```python
from build123d import *

# Parameters (mm, degrees)
SZKIC1_W                     = 100
SZKIC1_H                     = 100
DODANIE_WYCI_GNI_CIE1_DEPTH  = 40
SZKIC3_R                     = 22.5
WYTNIJ_WYCI_GNI_CIE1_DEPTH   = 41
SZKIC4_W                     = 100
SZKIC4_H                     = 10
DODANIE_WYCI_GNI_CIE2_DEPTH  = 30
DODANIE_WYCI_GNI_CIE3_DEPTH  = 10
DODANIE_WYCI_GNI_CIE4_DEPTH  = 10
DODANIE_WYCI_GNI_CIE5_DEPTH  = 10
SZKIC11_W                    = 15
SZKIC11_H                    = 50
DODANIE_WYCI_GNI_CIE6_DEPTH  = 70
SZKIC12_R                    = 15
DODANIE_WYCI_GNI_CIE7_DEPTH  = 125
SZKIC13_R                    = 15
DODANIE_WYCI_GNI_CIE8_DEPTH  = 30
DODANIE_WYCI_GNI_CIE9_DEPTH  = 10
ZAOKR_GLENIE1_R              = 20
SZKIC15_W                    = 50
SZKIC15_H                    = 185
DODANIE_WYCI_GNI_CIE10_DEPTH = 10
DODANIE_WYCI_GNI_CIE11_REACH = 52
SZKIC17_W                    = 50
SZKIC17_H                    = 30
SZKIC18_W                    = 100
SZKIC18_H                    = 100
DODANIE_WYCI_GNI_CIE12_DEPTH = 10
DODANIE_WYCI_GNI_CIE13_DEPTH = 10
WYTNIJ_WYCI_GNI_CIE2_REACH   = 202
SZKIC20_R                    = 5
SZKIC21_W                    = 10
SZKIC21_H                    = 25
DODANIE_WYCI_GNI_CIE14_DEPTH = 25
ZAOKR_GLENIE2_R              = 10
WYTNIJ_WYCI_GNI_CIE3_REACH   = 32
SZKIC22_R                    = 5


with BuildPart() as part:
    # Szkic1 → Dodanie-wyciągnięcie1 (new body)
    with BuildSketch(Plane.XY):
        Rectangle(SZKIC1_W, SZKIC1_H)
    extrude(amount=DODANIE_WYCI_GNI_CIE1_DEPTH)

    # Szkic3 → Wytnij-wyciągnięcie1 (cut, through all)
    with BuildSketch(Plane.XY.offset(40)):
        Circle(SZKIC3_R)
    extrude(amount=-WYTNIJ_WYCI_GNI_CIE1_DEPTH, mode=Mode.SUBTRACT)

    # Szkic4 → Dodanie-wyciągnięcie2 (add)
    with BuildSketch(Plane(origin=(0, 0, 0), x_dir=(-1, 0, 0), z_dir=(0, 0, -1))):
        with Locations((0, -45)):
            Rectangle(SZKIC4_W, SZKIC4_H)
    extrude(amount=DODANIE_WYCI_GNI_CIE2_DEPTH)

    # Szkic5 → Dodanie-wyciągnięcie3 (add)
    with BuildSketch(Plane.ZY.offset(50)):
        Polygon((-30, -40), (-250, 50), (0, 50), (0, -40), align=None)
    extrude(amount=-DODANIE_WYCI_GNI_CIE3_DEPTH)

    # Szkic6 → Dodanie-wyciągnięcie4 (add)
    with BuildSketch(Plane(origin=(50, 0, 0), x_dir=(0, 0, -1), z_dir=(1, 0, 0))):
        Polygon((30, -40), (250, 50), (0, 50), (0, -40), align=None)
    extrude(amount=-DODANIE_WYCI_GNI_CIE4_DEPTH)

    # Szkic7 → Dodanie-wyciągnięcie5 (add)
    with BuildSketch(Plane(origin=(0, 50, 0), x_dir=(1, 0, 0), z_dir=(0, 1, 0))):
        Polygon((40, 250), (-40, 250), (-40, 30), (-40, 0), (40, 0), align=None)
    extrude(amount=-DODANIE_WYCI_GNI_CIE5_DEPTH)

    # Szkic10 → Obrót1 (revolve)
    with BuildSketch(Plane(origin=(0, 0, -200), x_dir=(-1, 0, 0), z_dir=(0, 0, -1))):
        Polygon((0, 50), (0, 80), (-50, 50), align=None)
    revolve(axis=Axis((0, 50, -200), (0, 1, 0)))

    # Szkic11 → Dodanie-wyciągnięcie6 (add)
    with BuildSketch(Plane.XZ.offset(50)):
        with Locations((42.5, -5)):
            Rectangle(SZKIC11_W, SZKIC11_H)
    extrude(amount=DODANIE_WYCI_GNI_CIE6_DEPTH)

    # Szkic12 → Dodanie-wyciągnięcie7 (add)
    with BuildSketch(Plane.ZY.offset(-35)):
        with Locations((-5, -85)):
            Circle(SZKIC12_R)
    extrude(amount=DODANIE_WYCI_GNI_CIE7_DEPTH)

    # Szkic13 → Dodanie-wyciągnięcie8 (add)
    with BuildSketch(Plane.ZY.offset(50)):
        with Locations((-40, 0)):
            Circle(SZKIC13_R)
    extrude(amount=DODANIE_WYCI_GNI_CIE8_DEPTH)

    # Szkic14 → Dodanie-wyciągnięcie9 (add)
    with BuildSketch(Plane.ZY.offset(60)):
        Polygon((-69.010894517, 20.037063975), (-26.999775325, 36.163621704), (26.755417107, -103.87344227), (-15.255702085, -120), align=None)
    extrude(amount=DODANIE_WYCI_GNI_CIE9_DEPTH)

    # Zaokrąglenie1
    zaokr_glenie1_edges = [part.edges().sort_by_distance(p)[0] for p in [
        (-65, 20.037063975, -69.010894517),
        (-65, -120, -15.255702085),
        (-65, -103.87344227, 26.755417107),
        (-65, 36.163621704, -26.999775325),
        (42.5, -120, 20),
        (42.5, -120, -30),
    ]]
    fillet(zaokr_glenie1_edges, radius=ZAOKR_GLENIE1_R)

    # Szkic15 → Dodanie-wyciągnięcie10 (add)
    with BuildSketch(Plane.ZY.offset(90)):
        with Locations((-5, -27.5)):
            Rectangle(SZKIC15_W, SZKIC15_H)
    extrude(amount=DODANIE_WYCI_GNI_CIE10_DEPTH)

    # Szkic17 → Dodanie-wyciągnięcie11 (add, up to next)
    with BuildSketch(Plane.ZY.offset(50), mode=Mode.PRIVATE) as dodanie_wyci_gni_cie11_sk1:
        with Locations((-5, 50)):
            Rectangle(SZKIC17_W, SZKIC17_H)
    dodanie_wyci_gni_cie11_tool1 = extrude(dodanie_wyci_gni_cie11_sk1.sketch, amount=DODANIE_WYCI_GNI_CIE11_REACH, mode=Mode.PRIVATE) - part.part
    add(dodanie_wyci_gni_cie11_tool1.solids().sort_by_distance((-50, 50, -5))[0])

    # Szkic18 → Dodanie-wyciągnięcie12 (add)
    with BuildSketch(Plane.XY.offset(40)):
        with BuildLine():
            Line((70, 0), (121.10211367, 88.511457251))
            ThreePointArc((121.10211367, 88.511457251), (-150, 0), (121.10211367, -88.511457251))
            Line((121.10211367, -88.511457251), (70, 0))
        make_face()
        Rectangle(SZKIC18_W, SZKIC18_H, mode=Mode.SUBTRACT)
    extrude(amount=-DODANIE_WYCI_GNI_CIE12_DEPTH)

    # Szkic19 → Dodanie-wyciągnięcie13 (add)
    with BuildSketch(Plane(origin=(50, 0, 0), x_dir=(0, 0, -1), z_dir=(1, 0, 0))):
        Polygon((-30, 50), (-9.958560776, 84.617058134), (185, 50), align=None)
    extrude(amount=-DODANIE_WYCI_GNI_CIE13_DEPTH)

    # Szkic20 → Wytnij-wyciągnięcie2 (cut, up to next)
    with BuildSketch(Plane(origin=(50, 0, 0), x_dir=(0, 0, -1), z_dir=(1, 0, 0)), mode=Mode.PRIVATE) as wytnij_wyci_gni_cie2_sk1:
        with Locations((-4.958560776, 69.617058134)):
            Circle(SZKIC20_R)
    wytnij_wyci_gni_cie2_tool1 = extrude(wytnij_wyci_gni_cie2_sk1.sketch, amount=-WYTNIJ_WYCI_GNI_CIE2_REACH, mode=Mode.PRIVATE) & part.part
    add(wytnij_wyci_gni_cie2_tool1.solids().sort_by_distance((50, 69.617058, 4.958561))[0], mode=Mode.SUBTRACT)

    # Szkic21 → Dodanie-wyciągnięcie14 (add)
    with BuildSketch(Plane(origin=(50, 0, 0), x_dir=(0, 0, -1), z_dir=(1, 0, 0))):
        with Locations((-15, 7.5)):
            Rectangle(SZKIC21_W, SZKIC21_H)
        with Locations((-15, -37.5)):
            Rectangle(SZKIC21_W, SZKIC21_H)
    extrude(amount=DODANIE_WYCI_GNI_CIE14_DEPTH)

    # Zaokrąglenie2
    zaokr_glenie2_edges = [part.edges().sort_by_distance(p)[0] for p in [
        (45, 84.617058134, 9.958560776),
        (75, 20, 15),
        (75, -5, 15),
        (75, -25, 15),
        (75, -50, 15),
    ]]
    fillet(zaokr_glenie2_edges, radius=ZAOKR_GLENIE2_R)

    # Szkic22 → Wytnij-wyciągnięcie3 (cut, up to next)
    with BuildSketch(Plane(origin=(0, 0, 10), x_dir=(-1, 0, 0), z_dir=(0, 0, -1)), mode=Mode.PRIVATE) as wytnij_wyci_gni_cie3_sk1:
        with Locations((-63, 7.5)):
            Circle(SZKIC22_R)
    wytnij_wyci_gni_cie3_tool1 = extrude(wytnij_wyci_gni_cie3_sk1.sketch, amount=-WYTNIJ_WYCI_GNI_CIE3_REACH, mode=Mode.PRIVATE) & part.part
    add(wytnij_wyci_gni_cie3_tool1.solids().sort_by_distance((63, 7.5, 10))[0], mode=Mode.SUBTRACT)
    # Szkic22 → Wytnij-wyciągnięcie3 (cut, up to next)
    with BuildSketch(Plane(origin=(0, 0, 10), x_dir=(-1, 0, 0), z_dir=(0, 0, -1)), mode=Mode.PRIVATE) as wytnij_wyci_gni_cie3_sk2:
        with Locations((-63, -37.5)):
            Circle(SZKIC22_R)
    wytnij_wyci_gni_cie3_tool2 = extrude(wytnij_wyci_gni_cie3_sk2.sketch, amount=-WYTNIJ_WYCI_GNI_CIE3_REACH, mode=Mode.PRIVATE) & part.part
    add(wytnij_wyci_gni_cie3_tool2.solids().sort_by_distance((63, -37.5, 10))[0], mode=Mode.SUBTRACT)


solid = part.part
```
Design review of the part built by this model. Coordinates are the model's own, in mm. A direction names the side the tool comes from. Give positions to 0.01 mm unless a question says otherwise; leave off trailing zeros. Write each loop counter-clockwise with the first axis right and the second up, starting at its lowest first coordinate (ties: lowest second). Pieces come first, ordered by that corner, then holes. Notation, with made-up numbers: (71, 57) -> (128, 57) arc R33 ccw to (128, 92) -> close; hole circle Ø10 at (81, 37.5). An arc over 180 degrees is marked (long way). Answer in a Markdown table with one row per item.
(1) Consider section A-A (x = 97). State the section outline as (y, z) points, then the cut area to 3 significant figures.
Results:
| item | result |
|---|---|
| outline | (-114.42, 30) -> (-46.77, 30) -> (-46.77, 40) -> (-114.42, 40) -> close; (46.77, 30) -> (114.42, 30) -> (114.42, 40) -> (46.77, 40) -> close |
| area | 1,350 mm2 |
(2) Consider section B-B (z = -96). State the section outline as (x, y) points, then the cut area to 3 significant figures.
Results:
| item | result |
|---|---|
| outline | (-50, -13) -> (-40, -13) -> (-40, 40) -> (40, 40) -> (40, -13) -> (50, -13) -> (50, 65.8) -> (40, 65.8) -> (40, 50) -> (-50, 50) -> close |
| area | 2,220 mm2 |
(3) Clearance check with flat-ended pins moving along their axes: pin 1 (2.5 mm diameter, centred on y = 8, z = 15, fed in from +X); pin 2 (15 mm diameter, centred on x = -34, z = -233.5, fed in from +Y); pin 3 (10 mm diameter, centred on x = 5, y = -81, fed in from -Z). State where each tip first meets the part, or that it passes through.
Results:
| item | result |
|---|---|
| pin 1 | x = 75 |
| pin 2 | y = 55.86 |
| pin 3 | z = -20 |
(4) Mouldability with a two-part tool opening along Y and no side actions: class faces 6 (the conical face through (4.67, 74.79, -207.32)), 7 (the flat face through (-64.93, -33.136, -0.398)), 8 (the flat face through (15, -45, -30)), 9 (the flat face through (95.91, -44.88, 35.07)) as +Y half, -Y half, draft (parallel to the pull), parting line (faces both ways), or undercut.
Results:
| item | result |
|---|---|
| face 6 | +Y half |
| face 7 | undercut |
| face 8 | draft |
| face 9 | undercut |
(5) For faces 1 (the flat face through (38, 50, -240)), 2 (the flat face through (40, 43, -243)), 3 (the flat face through (57, 7, 10)), 4 (the flat face through (40, 60, -51)), 5 (the flat face through (17, 18, 0)), list the 3-axis set-ups (+Z, -Z, +X, -X, +Y, -Y) from which the entire face can be reached by the end or side of a thin tool; tool diameter is ignored.
Results:
| item | result |
|---|---|
| face 1 | -Z, +X, +Y |
| face 2 | -Z, +X, -Y |
| face 3 | -Z, +X, +Y, -Y |
| face 4 | +Y |
| face 5 | -Z |
(6) Consider section D-D (y = 103). State the section outline as (x, z) points.
Results:
| item | result |
|---|---|
| outline | (-109.05, 30) -> (109.05, 30) -> (109.05, 40) -> (-109.05, 40) -> close |
(7) To check wall thickness, follow probe 1 along Y at (x, z) = (63, 16); probe 2 along Y at (x, z) = (0, 19); probe 3 along Z at (x, y) = (-72.5, -84). State the ranges of each line that lie inside material, in increasing order.
Results:
| item | result |
|---|---|
| probe 1 | -50 to -42.5, -32.5 to -25, -5 to 2.5, 12.5 to 20 |
| probe 2 | -50 to -22.5, 22.5 to 50 |
| probe 3 | -19.97 to 9.97, 30 to 40 |
(8) Consider section C-C (z = -5). Count the separate pieces of the cut face and the enclosed holes in it, then the cut area to 3 significant figures.
Results:
| item | result |
|---|---|
| separate pieces | 1 |
| enclosed holes | 2 |
| area | 12,400 mm2 |
